Model file for the job. Use its own axes, mm. Face numbers are marked on the shaded views. A direction names the side the tool comes from. Round coordinates to 2 decimals unless told otherwise and drop trailing zeros. Order: outer loops, then holes, each group sorted by start corner. A loop starts at its lowest first (then second) coordinate and runs counter-clockwise, first axis right, second up. Notation, with made-up numbers: (-26, 29) -> (-3, 29) arc R21 ccw to (-3, 58) -> close; hole circle Ø11 at (61.5, 75). An arc over 180 degrees is marked (long way). Put each result on its own line as item: value. Start each with the question number.
Q1. 3-axis set-ups, long thin cutter, end or side, ignore diameter. For the marked faces 1, 2 and 3: which of +Z, -Z, +X, -X, +Y, -Y reach the whole face in a straight line?
Q2. Cut at D-D, the plane x = -24. List the corners of the cut face in (y, z), and give its area (3 significant figures).
Q3. Cut at B-B, the plane x = 10. List the corners of the cut face in (y, z), and give its area (3 significant figures).
Q4. Cut at C-C, the plane z = -10. List the corners of the cut face in (x, y).
Q5. Probe L1, parallel to X at y = 6.25, z = 10; L2, parallel to Z at x = 34, y = 6. List the from-to ranges inside material, lowest first.
Q6. Pull direction Z, two halves, no side cores. Call the marked faces 4, 5 and 6: released by +Z, released by -Z, zero draft, split by the parting line, or undercut.
Q7. Cut at A-A, the plane y = 13.5. List the corners of the cut face in (x, z).
Q8. Flat gauge pins, fed straight in: P1, Ø1.7, axis at y = 11.5, z = -9.5, coming from the +X side; P2, Ø3, axis at y = 13, z = -46.5, coming from the -X side; P3, Ø3, axis at y = 13.5, z = -49, coming from the +X side; P4, Ø2, axis at x = -5, z = 6, coming from the -Y side. Where does each tip first touch, or does it go through?
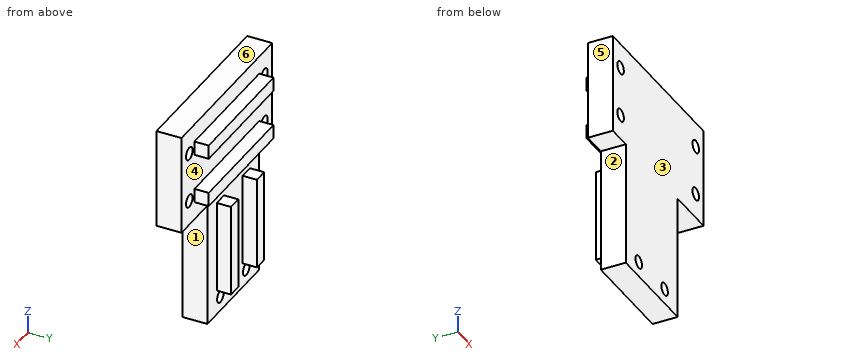
from build123d import *

# Parameters (mm, degrees)
SALIENTE_EXTRUIR1_DEPTH = 10
SALIENTE_EXTRUIR3_DEPTH = 100
CROQUIS5_W              = 40
CROQUIS5_H              = 50
SALIENTE_EXTRUIR5_DEPTH = 10
SALIENTE_EXTRUIR7_DEPTH = 47
CROQUIS13_W             = 59.276280914
CROQUIS13_H             = 44.398623438
CORTAR_EXTRUIR4_DEPTH   = 30
CROQUIS14_R             = 2.5
CORTAR_EXTRUIR5_DEPTH   = 16.7
CROQUIS15_W             = 10
CROQUIS15_H             = 40
CROQUIS15_W_2           = 40
CROQUIS15_H_2           = 10
CORTAR_EXTRUIR6_DEPTH   = 6.7


with BuildPart() as part:
    # Croquis1 → Saliente-Extruir1 (new body)
    with BuildSketch(Plane(origin=(0, 0, 0), x_dir=(1, 0, 0), z_dir=(0, 1, 0))):
        Polygon((20, 20), (-30, 20), (-30, -20), (40, -20), (70, -20), (70, 20), align=None)
    extrude(amount=SALIENTE_EXTRUIR1_DEPTH)

    # Croquis3 → Saliente-Extruir3 (add)
    with BuildSketch(Plane.ZY.offset(30)):
        Polygon((10, 10), (12.8, 10), (12.8, 15.7), (7.2, 15.7), (7.2, 10), align=None)
        Polygon((-10, 10), (-7.2, 10), (-7.2, 15.7), (-12.8, 15.7), (-12.8, 10), align=None)
    extrude(amount=-SALIENTE_EXTRUIR3_DEPTH)

    # Croquis5 → Saliente-Extruir5 (add)
    with BuildSketch(Plane(origin=(0, 10, 0), x_dir=(1, 0, 0), z_dir=(0, 1, 0))):
        with Locations((0, 45)):
            Rectangle(CROQUIS5_W, CROQUIS5_H)
    extrude(amount=-SALIENTE_EXTRUIR5_DEPTH)

    # Croquis7 → Saliente-Extruir7 (add)
    with BuildSketch(Plane(origin=(0, 0, -70), x_dir=(-1, 0, 0), z_dir=(0, 0, -1))):
        Polygon((-10, 10), (-12.8, 10), (-12.8, 15.7), (-7.2, 15.7), (-7.2, 10), align=None)
        Polygon((10, 10), (7.2, 10), (7.2, 15.7), (12.8, 15.7), (12.8, 10), align=None)
    extrude(amount=-SALIENTE_EXTRUIR7_DEPTH)

    # Croquis13 → Cortar-Extruir4 (cut)
    with BuildSketch(Plane(origin=(70, 0, 0), x_dir=(0, 0, -1), z_dir=(1, 0, 0))):
        Rectangle(CROQUIS13_W, CROQUIS13_H)
    extrude(amount=-CORTAR_EXTRUIR4_DEPTH, mode=Mode.SUBTRACT)

    # Croquis14 → Cortar-Extruir5 (cut, through all)
    with BuildSketch(Plane(origin=(0, 0, 0), x_dir=(-1, 0, 0), z_dir=(0, -1, 0))):
        with Locations((-34, -10)):
            Circle(CROQUIS14_R)
        with Locations((-34, 10)):
            Circle(CROQUIS14_R)
        with Locations((24, -10)):
            Circle(CROQUIS14_R)
        with Locations((24, 10)):
            Circle(CROQUIS14_R)
        with Locations((10, 64)):
            Circle(CROQUIS14_R)
        with Locations((-10, 64)):
            Circle(CROQUIS14_R)
    extrude(amount=-CORTAR_EXTRUIR5_DEPTH, mode=Mode.SUBTRACT)

    # Croquis15 → Cortar-Extruir6 (cut, through all)
    with BuildSketch(Plane(origin=(0, 10, 0), x_dir=(1, 0, 0), z_dir=(0, 1, 0))):
        with Locations((35, 0)):
            Rectangle(CROQUIS15_W, CROQUIS15_H)
        with Locations((-25, 0)):
            Rectangle(CROQUIS15_W, CROQUIS15_H)
        with Locations((0, 65)):
            Rectangle(CROQUIS15_W_2, CROQUIS15_H_2)
    extrude(amount=CORTAR_EXTRUIR6_DEPTH, mode=Mode.SUBTRACT)


solid = part.part
Ans:
1. face 1: -Z, +X, +Y, -Y
1. face 2: -Z, -X, +Y, -Y
1. face 3: +Z, -Z, +X, -X, -Y
2. outline: (0, -20) -> (10, -20) -> (10, -12.5) -> (0, -12.5) -> close; (0, -7.5) -> (10, -7.5) -> (10, 7.5) -> (0, 7.5) -> close; (0, 12.5) -> (10, 12.5) -> (10, 20) -> (0, 20) -> close
2. area: 300 mm^2
3. outline: (0, -70) -> (10, -70) -> (10, -66.5) -> (0, -66.5) -> close; (0, -61.5) -> (10, -61.5) -> (10, -60) -> (15.7, -60) -> (15.7, -23) -> (10, -23) -> (10, -12.8) -> (15.7, -12.8) -> (15.7, -7.2) -> (10, -7.2) -> (10, 7.2) -> (15.7, 7.2) -> (15.7, 12.8) -> (10, 12.8) -> (10, 20) -> (0, 20) -> close
3. area: 1,120 mm^2
4. outline: (-30, 0) -> (-26.5, 0) -> (-26.5, 10) -> (-30, 10) -> close; (-21.5, 0) -> (31.5, 0) -> (31.5, 10) -> (30, 10) -> (30, 15.7) -> (-20, 15.7) -> (-20, 10) -> (-21.5, 10) -> close; (36.5, 0) -> (40, 0) -> (40, 10) -> (36.5, 10) -> close
5. L1: x = -30 to -26.5, -21.5 to 31.5, 36.5 to 40
5. L2: z = -20 to -12.5, -7.5 to 7.5, 12.5 to 20
6. face 4: undercut
6. face 5: zero draft
6. face 6: released by +Z
7. outline: (-20, -12.8) -> (30, -12.8) -> (30, -7.2) -> (-20, -7.2) -> close; (-20, 7.2) -> (30, 7.2) -> (30, 12.8) -> (-20, 12.8) -> close; (-12.8, -60) -> (-7.2, -60) -> (-7.2, -23) -> (-12.8, -23) -> close; (7.2, -60) -> (12.8, -60) -> (12.8, -23) -> (7.2, -23) -> close
8. P1: stops at x = 30
8. P2: stops at x = -12.8
8. P3: stops at x = 12.8
8. P4: stops at y = 0
